```python
from build123d import *

# Parameters (mm, degrees)
F1_DEPTH = 63.5
F3_DEPTH = 57.15


with BuildPart() as f1:
    # F0 (on Front) → F1 (new body)
    with BuildSketch(Plane.XZ):
        with BuildLine():
            Line((393.824851, 57.15), (304.8, 57.15))
            Line((304.8, 57.15), (304.8, -57.15))
            Line((304.8, -57.15), (393.404788, -48.661999))
            ThreePointArc((393.404788, -48.661999), (411.620709, -51.38959), (426.428465, -62.34358))
            ThreePointArc((426.428465, -62.34358), (455.726477, -87.137442), (491.847598, -100.113334))
            ThreePointArc((491.847598, -100.113334), (508.73791, -107.460232), (520.208033, -121.871887))
            Line((520.208033, -121.871887), (557.159603, -202.849885))
            Line((557.159603, -202.849885), (656.146307, -145.699885))
            Line((656.146307, -145.699885), (611.633881, -68.602102))
            ThreePointArc((611.633881, -68.602102), (606.610921, -52.042385), (609.430848, -34.968945))
            ThreePointArc((609.430848, -34.968945), (611.924023, 41.045153), (563.676477, 99.837442))
            ThreePointArc((563.676477, 99.837442), (488.637088, 112.224898), (424.053536, 72.058696))
            ThreePointArc((424.053536, 72.058696), (410.677467, 61.079847), (393.824851, 57.15))
        make_face()
    extrude(amount=F1_DEPTH)


with BuildPart() as f3:
    # F2 (on face) → F3 (new body)
    with BuildSketch(Plane.XZ.offset(63.5)):
        with BuildLine():
            Line((293.525537, -51.85098), (419.194066, -39.812414))
            ThreePointArc((419.194066, -39.812414), (458.901477, -81.638181), (514.977359, -95.112925))
            Line((514.977359, -95.112925), (570.314071, -216.38128))
            Line((570.314071, -216.38128), (656.146307, -158.399885))
            Line((656.146307, -158.399885), (593.876602, -50.545592))
            ThreePointArc((593.876602, -50.545592), (560.501477, 94.338181), (418.340887, 50.8))
            Line((418.340887, 50.8), (288.119435, 50.8))
            Line((288.119435, 50.8), (293.525537, -51.85098))
        make_face()
    extrude(amount=-F3_DEPTH)


with BuildPart() as f1_1:
    add(f1.part)

    # F4: cut F3
    add(f3.part, mode=Mode.SUBTRACT)


solid = f1_1.part
```
CAD build for the part. Positions are in the model's coordinates, mm. A direction names the side the tool comes from. Round coordinates to 2 decimals unless told otherwise and drop trailing zeros. Order: outer loops, then holes, each group sorted by start corner. A loop starts at its lowest first (then second) coordinate and runs counter-clockwise, first axis right, second up.
Item 1: Saw through at C-C on x = 400.5. Write the cut outline in (y, z), then the cut area to 3 significant figures.
Item 2: Saw through at D-D on z = -117.5. Write the cut outline in (x, y), then the cut area to 3 significant figures.
Item 3: Pin check, flat tips, straight feed: pin 1 (10 mm diameter, centred on y = -19.5, z = 78, fed in from -X); pin 2 (6 mm diameter, centred on x = 505, y = -42.5, fed in from +Z); pin 3 (3 mm diameter, centred on x = 379, y = -50.5, fed in from -Z). Stop position of each tip, or through.
Item 4: Saw through at B-B on z = 6.35. Write the cut outline in (x, y), then the cut area to 3 significant figures.
Item 5: Saw through at A-A on y = -31.5. Write the cut outline in (x, z), then the cut area to 3 significant figures.
Item 6: Tool access for faces 4 (the face through (562.51, -35.325, 93.148)), 5 (the face through (362, -35, 50.8)), 6 (the face through (350, -31, 57.15)): list every direction of +Z, -Z, +X, -X, +Y, -Y with a clear straight run to the whole face (end or side of a thin tool).
Item 7: Mould opens along X. For faces 1 (the face through (304.8, -6, 9)), 2 (the face through (452.2, -63.5, -84.7)), 3 (the face through (348.482, -31.306, -52.965)) say: pulls with the +X half, pulls with the -X half, needs draft (parallel to the pull), parting line crosses it, or undercut.
Item 8: Probe line 1 along Y through (x, z) = (574.5, 31); line 2 along Z through (x, y) = (489, -42); line 3 along X through (y, z) = (-32, 53). List the from-to ranges inside material, lowest first.
Reported:
1. outline: (-63.5, -48.65) - (0, -48.65) - (0, 57.74) - (-63.5, 57.74) - (-63.5, 50.8) - (-6.35, 50.8) - (-6.35, -41.6) - (-63.5, -41.6) - close
1. area: 1,470 mm2
2. outline: (517.86, -63.5) - (525.19, -63.5) - (525.19, -6.35) - (632.53, -6.35) - (632.53, -63.5) - (639.87, -63.5) - (639.87, 0) - (517.86, 0) - close
2. area: 1,610 mm2
3. pin 1: stops at x = 424.78
3. pin 2: stops at z = 114.29
3. pin 3: stops at z = -50.19
4. outline: (304.8, -6.35) - (611.3, -6.35) - (611.3, -63.5) - (617.65, -63.5) - (617.65, 0) - (304.8, 0) - close
4. area: 2,350 mm2
5. outline: (304.8, -57.15) - (393.4, -48.66) arc R38.1 cw to (426.43, -62.34) arc R107.95 ccw to (491.85, -100.11) arc R38.1 cw to (520.21, -121.87) - (557.16, -202.85) - (562.68, -199.66) - (514.98, -95.11) arc R101.6 cw to (419.19, -39.81) - (304.8, -50.77) - close; (304.8, 50.8) - (418.34, 50.8) arc R101.6 cw (long way) to (593.88, -50.55) - (650.65, -148.87) - (656.15, -145.7) - (611.63, -68.6) arc R38.1 cw to (609.43, -34.97) arc R107.95 ccw to (563.68, 99.84) arc R107.95 ccw to (424.05, 72.06) arc R38.1 cw to (393.82, 57.15) - (304.8, 57.15) - close
5. area: 6,020 mm2
6. face 4: -Y
6. face 5: -X, -Y
6. face 6: +Z, -X, +Y, -Y
7. face 1: pulls with the -X half
7. face 2: needs draft
7. face 3: undercut
8. line 1: y = -6.35 to 0
8. line 2: z = -99.6 to -93.12, 105.82 to 112.3
8. line 3: x = 304.8 to 419.44, 599.96 to 607.05
